Input: part model. Units: mm. Frame: model coordinates. Face numbers are marked on the shaded views. A direction names the side the tool comes from. Coordinates: 2 decimals unless noted, no trailing zeros. Order: outer loops, then holes, each group sorted by start corner. A loop starts at its lowest first (then second) coordinate and runs counter-clockwise, first axis right, second up. Notation, with made-up numbers: (-27, -33.75) -> (24, -33.75) arc R29 ccw to (24, -9.75) -> close; hole circle Ø8 at (71, 29). An arc over 180 degrees is marked (long way). One line per question, with ' | ' between items.
```python
from build123d import *

# Parameters (mm, degrees)
F0_W      = 35
F0_H      = 45
F1_DEPTH  = 4.5
F2_R      = 2
F3_DEPTH  = 10
F4_W      = 35
F4_H      = 10
F5_DEPTH  = 10
F6_R      = 3
F7_DEPTH  = 6
F8_W      = 35
F8_H      = 4.5
F9_DEPTH  = 2
F10_W     = 12
F10_H     = 25
F11_DEPTH = 14.501
F12_R     = 1.5
F13_DEPTH = 23.001
F14_W     = 35
F14_H     = 6
F15_DEPTH = 4.501
F16_W     = 35
F16_H     = 4.5
F17_DEPTH = 1


with BuildPart() as f1:
    # F0 (on Front) → F1 (new body)
    with BuildSketch(Plane.XZ):
        with Locations((0, 2.5)):
            Rectangle(F0_W, F0_H)
    extrude(amount=F1_DEPTH)

    # F2 (on face) → F3 (cut)
    with BuildSketch(Plane.XZ.offset(4.5)):
        with Locations((12.5, -15)):
            Circle(F2_R)
        with Locations((-12.5, -15)):
            Circle(F2_R)
        with Locations((-12.5, -7)):
            Circle(F2_R)
        with Locations((12.5, -7)):
            Circle(F2_R)
    extrude(amount=-F3_DEPTH, mode=Mode.SUBTRACT)

    # F4 (on face) → F5 (join)
    with BuildSketch(Plane.XZ.offset(4.5)):
        with Locations((0, 20)):
            Rectangle(F4_W, F4_H)
    extrude(amount=F5_DEPTH)

    # F6 (on face) → F7 (cut)
    with BuildSketch(Plane(origin=(0, 0, 15), x_dir=(1, 0, 0), z_dir=(0, 0, -1))):
        with Locations((0, 9.5)):
            Circle(F6_R)
    extrude(amount=-F7_DEPTH, mode=Mode.SUBTRACT)

    # F8 (on face) → F9 (cut)
    with BuildSketch(Plane(origin=(0, 0, -20), x_dir=(1, 0, 0), z_dir=(0, 0, -1))):
        with Locations((0, 2.25)):
            Rectangle(F8_W, F8_H)
    extrude(amount=-F9_DEPTH, mode=Mode.SUBTRACT)

    # F10 (on face) → F11 (cut, through all)
    with BuildSketch(Plane.XZ.offset(14.5)):
        with Locations((-11.5, 12.5)):
            Rectangle(F10_W, F10_H)
        with Locations((11.5, 12.5)):
            Rectangle(F10_W, F10_H)
    extrude(amount=-F11_DEPTH, mode=Mode.SUBTRACT)

    # F12 (on face) → F13 (cut, through all)
    with BuildSketch(Plane.YZ.offset(5.5)):
        with Locations((-9.5, 18)):
            Circle(F12_R)
    extrude(amount=-F13_DEPTH, mode=Mode.SUBTRACT)

    # F14 (on face) → F15 (cut, through all)
    with BuildSketch(Plane.XZ.offset(4.5)):
        with Locations((0, -15)):
            Rectangle(F14_W, F14_H)
    extrude(amount=-F15_DEPTH, mode=Mode.SUBTRACT)

    # F16 (on face) → F17 (cut)
    with BuildSketch(Plane(origin=(0, 0, -12), x_dir=(1, 0, 0), z_dir=(0, 0, -1))):
        with Locations((0, 2.25)):
            Rectangle(F16_W, F16_H)
    extrude(amount=-F17_DEPTH, mode=Mode.SUBTRACT)


solid = f1.part
```
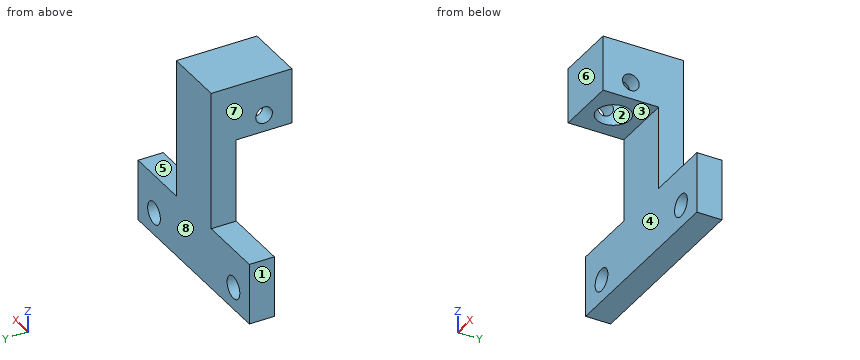
1. Access query for the marked faces 4, 5, 6, 7 and 8. Directions: +Z, -Z, +X, -X, +Y, -Y. A direction counts if a zero-diameter tool reaches every point of the face in a straight line with its end or side. Return the directions, or none.
Recorded:
face 4: -Z, +X, -X, -Y | face 5: +Z, +X, +Y, -Y | face 6: +Z, -Z, +X, -X, -Y | face 7: +Z, -X, +Y, -Y | face 8: +Z, -Z, +X, -X, +Y
2. Pin query (flat end, axial travel): pin 1 Ø4.5 at (x, z) = (12.5, -7) entering from -Y; pin 2 Ø3.5 at (x, y) = (10, -1.5) entering from +Z; pin 3 Ø4 at (y, z) = (-9.5, 18) entering from +X. Return the tip coordinate at first contact, or that it passes through.
Recorded:
pin 1: stops at y = -4.5 | pin 2: stops at z = 0 | pin 3: stops at x = 5.5
3. Cut plane A-A, the plane x = -3.5. Return loops of the section in (y, z).
Recorded:
outline: (-14.5, 15) -> (-4.5, 15) -> (-4.5, -11) -> (0, -11) -> (0, 25) -> (-14.5, 25) -> close; hole circle Ø3 at (-9.5, 18)
4. Cut plane D-D, the plane x = -12.5. Return loops of the section in (y, z).
Recorded:
outline: (-4.5, -11) -> (0, -11) -> (0, -9) -> (-4.5, -9) -> close; (-4.5, -5) -> (0, -5) -> (0, 0) -> (-4.5, 0) -> close
5. Cut plane C-C, the plane z = -7. Return loops of the section in (x, y).
Recorded:
outline: (-17.5, -4.5) -> (-14.5, -4.5) -> (-14.5, 0) -> (-17.5, 0) -> close; (-10.5, -4.5) -> (10.5, -4.5) -> (10.5, 0) -> (-10.5, 0) -> close; (14.5, -4.5) -> (17.5, -4.5) -> (17.5, 0) -> (14.5, 0) -> close
6. Mould query, pull axis X, two halves, no side actions, for the marked faces 1, 2 and 3. Classes: released by +X, released by -X, zero draft, split by the parting line, or undercut.
Recorded:
face 1: released by -X | face 2: undercut | face 3: zero draft
7. Ray query, line 1 (Y direction, x = 0, z = 18); line 2 (Z direction, x = -12.5, y = -2.8); line 3 (X direction, y = -3.25, z = -6). Return the intervals inside material, ascending. Write a range as [from, to].
Recorded:
line 1: y = [-14.5, -12.5], [-6.5, 0] | line 2: z = [-11, -9], [-5, 0] | line 3: x = [-17.5, -14.23], [-10.77, 10.77], [14.23, 17.5]
8. Cut plane B-B, the plane z = 18. Return loops of the section in (x, y).
Recorded:
outline: (-5.5, -14.5) -> (5.5, -14.5) -> (5.5, -11) -> (2.6, -11) arc R3 cw to (-2.6, -11) -> (-5.5, -11) -> close; (-5.5, -8) -> (-2.6, -8) arc R3 cw to (2.6, -8) -> (5.5, -8) -> (5.5, 0) -> (-5.5, 0) -> close
